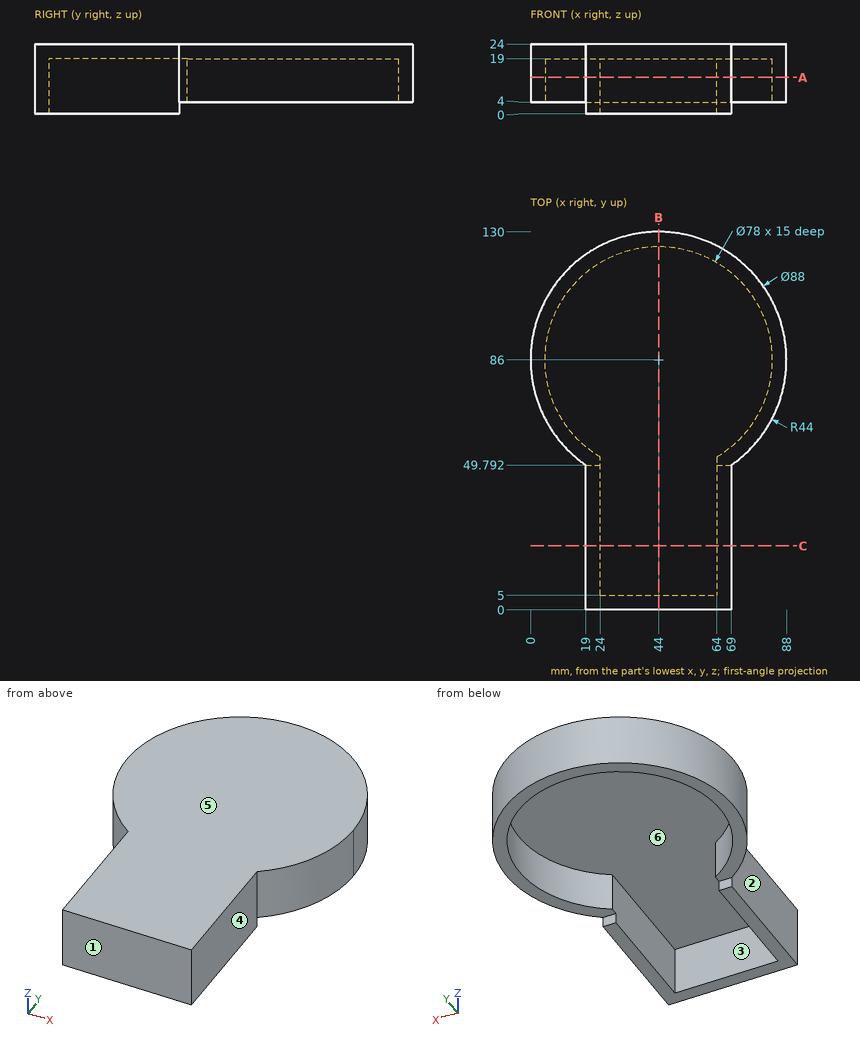
Job drawing, mm, ordinate dimensions from the low corner. One solid piece. A direction names the side the tool comes from. Give positions to 0.01 mm unless a question says otherwise; leave off trailing zeros. Order: outer loops, then holes, each group sorted by start corner. A loop starts at its lowest first (then second) coordinate and runs counter-clockwise, first axis right, second up. Notation, with made-up numbers: (43.5, -39) - (89.5, -39) arc R20 ccw to (89.5, -25) - close; hole circle Ø5 at (1, 33). An arc over 180 degrees is marked (long way). Return JSON: item names as keys, results as strings.
1) Probe line 1 (Y direction, x = 44, z = 9.25); line 2 (X direction, y = 86, z = 10.75); line 3 (X direction, y = 24, z = 12.25). List the from-to ranges inside material, lowest first. Write a range as from..to.
Geometry says:
{"line 1": "0..5, 125..130", "line 2": "0..5, 83..88", "line 3": "19..24, 64..69"}
2) Cut at A-A, the plane z = 12.5. Give the cut face in (x, y), plus the area to 3 significant figures.
Geometry says:
{"outline": "(19, 0) - (69, 0) - (69, 49.79) arc R44 ccw (long way) to (19, 49.79) - close; hole (24, 5) - (64, 5) - (64, 52.52) arc R39 ccw (long way) to (24, 52.52) - close", "area": "1,780 mm²"}
3) Flat gauge pins, fed straight in: P1, Ø2, axis at x = 16.5, z = 13, coming from the +Y side (1 decimal); P2, Ø4, axis at x = 53, y = 32.5, coming from the -Z side; P3, Ø4.5, axis at x = 21.5, z = 1.5, coming from the +Y side. Where does each tip first touch, or does it go through?
Geometry says:
{"P1": "y = 121.1", "P2": "z = 19", "P3": "y = 49.79"}
4) Cut at B-B, the plane x = 44. Give the cut face in (y, z).
Geometry says:
{"outline": "(0, 0) - (5, 0) - (5, 19) - (125, 19) - (125, 4) - (130, 4) - (130, 24) - (0, 24) - close"}
5) 3-axis set-ups, long thin cutter, end or side, ignore diameter. For the marked faces 1, 2 and 3: which of +Z, -Z, +X, -X, +Y, -Y reach the whole face in a straight line?
Geometry says:
{"face 1": "+Z, -Z, +X, -X, -Y", "face 2": "+Z, -Z, -X, -Y", "face 3": "-Z"}
6) Pull direction X, two halves, no side cores. Call the marked faces 4, 5 and 6: pulls with the +X half, pulls with the -X half, needs draft (parallel to the pull), parting line crosses it, or undercut.
Geometry says:
{"face 4": "pulls with the +X half", "face 5": "needs draft", "face 6": "undercut"}
7) Cut at C-C, the plane y = 22. Give the cut face in (x, z).
Geometry says:
{"outline": "(19, 0) - (24, 0) - (24, 19) - (64, 19) - (64, 0) - (69, 0) - (69, 24) - (19, 24) - close"}
